Could you check a few things on this drawing? It's one solid part, dimensions in mm from its lowest x, y, z. A direction names the side the tool comes from. Coordinates: 2 decimals unless noted, no trailing zeros. Order: outer loops, then holes, each group sorted by start corner. A loop starts at its lowest first (then second) coordinate and runs counter-clockwise, first axis right, second up.
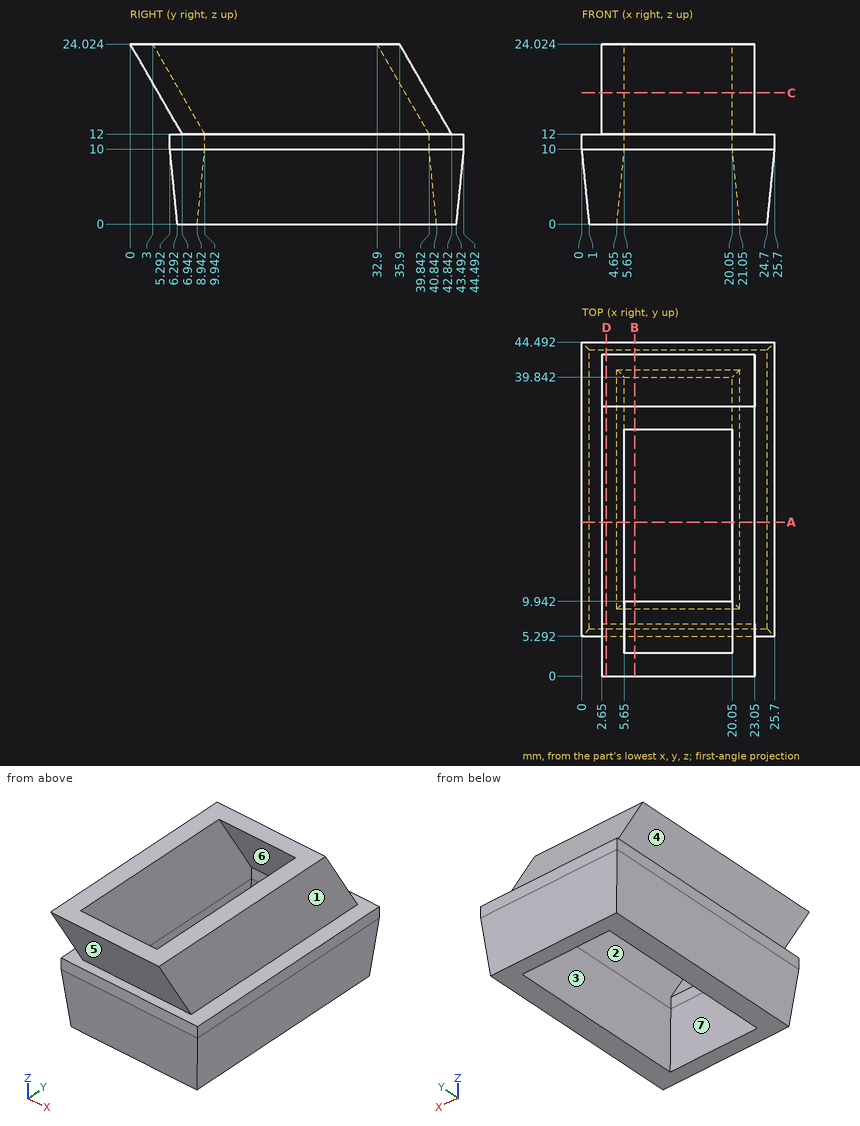
1. Please list where these lines run through material, in increasing order: probe 1 along X at (y, z) = (18, 13); probe 2 along Z at (x, y) = (23.5, 29.5); probe 3 along X at (y, z) = (38, 10.5).
Completed:
probe 1: x = 2.65 to 5.65, 20.05 to 23.05
probe 2: z = 0 to 12
probe 3: x = 0 to 5.65, 20.05 to 25.7
2. Imagine slicing it at C-C on z = 17.5. Please give me the cut outline in (x, y), then the cut area to 3 significant figures.
Completed:
outline: (2.65, 3.77) - (23.05, 3.77) - (23.05, 39.67) - (2.65, 39.67) - close; hole (5.65, 6.77) - (20.05, 6.77) - (20.05, 36.67) - (5.65, 36.67) - close
area: 302 mm2
3. Imagine slicing it at B-B on x = 7. Please give me the cut outline in (y, z), then the cut area to 3 significant figures.
Completed:
outline: (0, 24.02) - (6.94, 12) - (5.29, 12) - (5.29, 10) - (6.29, 0) - (8.94, 0) - (9.94, 10) - (9.94, 12) - (3, 24.02) - close; (32.9, 24.02) - (39.84, 12) - (39.84, 10) - (40.84, 0) - (43.49, 0) - (44.49, 10) - (44.49, 12) - (42.84, 12) - (35.9, 24.02) - close
area: 164 mm2
4. Imagine slicing it at A-A on y = 20.5. Please give me the cut outline in (x, z), then the cut area to 3 significant figures.
Completed:
outline: (0, 10) - (1, 0) - (4.65, 0) - (5.65, 10) - (5.65, 24.02) - (2.65, 24.02) - (2.65, 12) - (0, 12) - close; (20.05, 10) - (21.05, 0) - (24.7, 0) - (25.7, 10) - (25.7, 12) - (23.05, 12) - (23.05, 24.02) - (20.05, 24.02) - close
area: 188 mm2
5. Thinking about a two-plate mould opening in X: for the marked faces 4, 5, 6 and 7, which applies, pulls with the +X half, pulls with the -X half, needs draft (parallel to the pull), parting line crosses it, or undercut?
Completed:
face 4: pulls with the -X half
face 5: needs draft
face 6: undercut
face 7: undercut
6. I'm going to push flat-ended pins straight in: pin 1 (3 mm diameter, centred on x = 17.5, y = 24, fed in from -Z); pin 2 (3.5 mm diameter, centred on y = 24.5, z = 17.5, fed in from -X); pin 3 (13 mm diameter, centred on y = 23, z = 17, fed in from +X); pin 4 (1.6 mm diameter, centred on x = 11, z = 10.5, fed in from -Y). Where does each tip first touch, or does it pass through?
Completed:
pin 1: passes through
pin 2: stops at x = 2.65
pin 3: stops at x = 25.7
pin 4: stops at y = 5.29
7. On a 3-axis mill with a long thin cutter (end or side, diameter ignored), from which of +Z, -Z, +X, -X, +Y, -Y can I reach the whole of each face in a straight line? I mean the marked faces 1, 2 and 3. Say none if no direction works.
Completed:
face 1: +Z, +X, +Y, -Y
face 2: none
face 3: -Z
8. Imagine slicing it at D-D on x = 3.25. Please give me the cut outline in (y, z).
Completed:
outline: (0, 24.02) - (6.94, 12) - (5.29, 12) - (5.29, 10) - (6.29, 0) - (43.49, 0) - (44.49, 10) - (44.49, 12) - (42.84, 12) - (35.9, 24.02) - close
